```python
from build123d import *

# Parameters (mm, degrees)
BOSS_EXTRUDE1_DEPTH = 160
SKETCH4_W           = 3.229565218
SKETCH4_H           = 38.29
SKETCH4_W_2         = 3.229565217
CUT_EXTRUDE1_DEPTH  = 174.405056443


with BuildPart() as part:
    # Sketch1 → Boss-Extrude1 (new body)
    with BuildSketch(Plane.XY):
        Polygon((-49.44, -45), (-49.44, 0), (49.44, 0), (49.44, -45), (45.14, -45), (45.14, -6.71), (37.14, -6.71), (37.14, -45), (-37.14, -45), (-37.14, -6.71), (-45.14, -6.71), (-45.14, -45), align=None)
    extrude(amount=-BOSS_EXTRUDE1_DEPTH)

    # Sketch4 → Cut-Extrude1 (cut, through all)
    with BuildSketch(Plane.XY):
        with Locations((-32.295652174, -25.855)):
            Rectangle(SKETCH4_W, SKETCH4_H)
        with Locations((-25.836521739, -25.855)):
            Rectangle(SKETCH4_W, SKETCH4_H)
        with Locations((-19.377391305, -25.855)):
            Rectangle(SKETCH4_W_2, SKETCH4_H)
        with Locations((-12.91826087, -25.855)):
            Rectangle(SKETCH4_W_2, SKETCH4_H)
        with Locations((-6.459130435, -25.855)):
            Rectangle(SKETCH4_W_2, SKETCH4_H)
        with Locations((0, -25.855)):
            Rectangle(SKETCH4_W, SKETCH4_H)
        with Locations((6.459130435, -25.855)):
            Rectangle(SKETCH4_W_2, SKETCH4_H)
        with Locations((12.91826087, -25.855)):
            Rectangle(SKETCH4_W_2, SKETCH4_H)
        with Locations((19.377391305, -25.855)):
            Rectangle(SKETCH4_W_2, SKETCH4_H)
        with Locations((25.836521739, -25.855)):
            Rectangle(SKETCH4_W, SKETCH4_H)
        with Locations((32.295652174, -25.855)):
            Rectangle(SKETCH4_W, SKETCH4_H)
    extrude(amount=-CUT_EXTRUDE1_DEPTH, mode=Mode.SUBTRACT)


solid = part.part
```
Verification items for the finished model (mm, model axes). A direction names the side the tool comes from. Round coordinates to 2 decimals unless told otherwise and drop trailing zeros. Loops run counter-clockwise (first coordinate to the right, second up) from the corner with the lowest first, then second, coordinate; pieces in that order, holes last. Notation, with made-up numbers: (-29.5, 56) -> (25.5, 56) arc R11 ccw to (25.5, 77) -> close; hole circle Ø7 at (23.25, 77). An arc over 180 degrees is marked (long way). Answer as a JSON object with one key per item and string values.
Q1. Section check B-B (x = 42). Record the boundary of the cut face in (y, z).
Data:
{"outline": "(-6.71, -160) -> (0, -160) -> (0, 0) -> (-6.71, 0) -> close"}
Q2. Scan line: line 1 (Y direction, x = 14, z = -129). Record every from-to range of solid material in increasing order. Write a range as from..to.
Data:
{"line 1": "y = -6.71..0"}
Q3. Section check A-A (y = -18). State how many separate pieces and enclosed holes the cut face has, then the cut area to 3 significant figures.
Data:
{"separate pieces": "14", "enclosed holes": "0", "area": "7,580 mm2"}
Q4. Go/stop test with a flat-tipped pin: P1, Ø1.6, axis at x = 26, z = -62, coming from the -Y side. Record where the tip stops, or that it passes through.
Data:
{"P1": "stops at y = -6.71"}
Q5. Access from +Z, -Z, +X, -X, +Y, -Y to the whole of each face (thin tool, end or side, straight path). Record for faces 1 (the flat face through (-33.91, -26, -79)), 2 (the flat face through (47, -45, -79)).
Data:
{"face 1": "+Z, -Z, -Y", "face 2": "+Z, -Z, +X, -X, -Y"}
